Autodesk Inventor part; units mm, degrees
ref_plane "YZ Plane" through (0, 0, 0) normal (1, 0, 0) x (0, 1, 0)
ref_plane "XZ Plane" through (0, 0, 0) normal (0, 1, 0) x (-1, 0, 0)
ref_plane "XY Plane" through (0, 0, 0) normal (0, 0, 1) x (1, 0, 0)
sketch "Sketch1" plane through (0, 0, 0) normal (0, 0, 1) x (1, 0, 0)
  line L0 (-61.3765, 63.5) -> (14.8235, 63.5)
  line L1 (52.9235, 25.4) -> (52.9235, 0)
  line L2 (52.9235, 0) -> (-61.3765, 0)
  line L3 (-61.3765, 0) -> (-61.3765, 63.5)
  line L4 (52.9235, 25.4) -> (14.8235, 25.4)
  line L5 (14.8235, 25.4) -> (14.8235, 63.5)
  point P0 (0, 0)
  dimension "d0" = 38.1
  dimension "d1" = 76.2
  dimension "d2" = 38.1
  dimension "d3" = 114.3
  dimension "d4" = 63.5
  dimension "d5" = 25.4
extrude "Extrusion1" add sketch "Sketch1" along normal blind 12.7
sketch "Sketch2" plane through (0, 0, 12.7) normal (0, 0, 1) x (1, 0, 0)
  line L0 (-61.3765, 0) -> (52.9235, 0)
  line L1 (-61.3765, 63.5) -> (-61.3765, 0)
  line L2 (52.9235, 0) -> (-61.3765, 0)
  line L3 (-61.3765, 0) -> (-61.3765, 12.7)
  line L4 (-61.3765, 12.7) -> (52.9235, 12.7)
  line L5 (52.9235, 12.7) -> (52.9235, 0)
  point P0 (0, 0)
  dimension "d8" = 12.7
extrude "Extrusion2" add sketch "Sketch2" along normal blind 12.7
sketch "Sketch3" plane through (0, 0, 0) normal (0, 0, -1) x (-1, 0, 0)
  line L0 (61.3765, 63.5) -> (61.3765, 12.7)
  line L1 (-14.8235, 25.4) -> (-14.8235, 63.5)
  line L2 (61.3765, 63.5) -> (-14.8235, 63.5)
  line L3 (-14.8235, 63.5) -> (-14.8235, 38.1)
  line L4 (-14.8235, 38.1) -> (61.3765, 38.1)
  line L5 (61.3765, 38.1) -> (61.3765, 63.5)
  point P0 (0, 0)
  dimension "d11" = 25.4
extrude "Extrusion3" add sketch "Sketch3" along normal blind 25.4
Could you check a few things on this model? Use its own coordinates, in mm. A direction names the side the tool comes from. Round coordinates to 2 decimals unless told otherwise and drop trailing zeros. Write each loop counter-clockwise with the first axis right and the second up, starting at its lowest first coordinate (ties: lowest second). Pieces come first, ordered by that corner, then holes. Notation, with made-up numbers: (10, 54) -> (63, 54) arc R29 ccw to (63, 87) -> close; hole circle Ø10 at (32.25, 17). An arc over 180 degrees is marked (long way). Use a Markdown table: item, result.
1. Please list where these lines run through material, in increasing order: probe 1 along Z at (x, y) = (-38, 60); probe 2 along Z at (x, y) = (-32, 21); probe 3 along X at (y, z) = (54, 2.5).
Answer key:
| item | result |
|---|---|
| probe 1 | z = -25.4 to 12.7 |
| probe 2 | z = 0 to 12.7 |
| probe 3 | x = -61.38 to 14.82 |
2. For pin 1 Ø2 at (x, y) = (32.5, 20.5) entering from +Z; pin 2 Ø19 at (y, z) = (46, -7) entering from +X; pin 3 Ø2 at (x, z) = (4, 8.5) entering from -Y; pin 4 Ø12.5 at (x, z) = (-24, -10) entering from -Y, each with a flat end and sliding along its axis, tell me the tip position at first contact or that it passes through.
Answer key:
| item | result |
|---|---|
| pin 1 | stops at z = 12.7 |
| pin 2 | stops at x = 14.82 |
| pin 3 | stops at y = 0 |
| pin 4 | stops at y = 38.1 |
3. If we section it at A-A (x = -30): List the corners of the cut face in (y, z) for me, then the cut area to 3 significant figures.
Answer key:
| item | result |
|---|---|
| outline | (0, 0) -> (38.1, 0) -> (38.1, -25.4) -> (63.5, -25.4) -> (63.5, 12.7) -> (12.7, 12.7) -> (12.7, 25.4) -> (0, 25.4) -> close |
| area | 1,610 mm^2 |
4. Which directions (+Z, -Z, +X, -X, +Y, -Y) give clear straight access to the entire face, cutting with the end or side of a thin tool? Please do faces 1 (the face through (14.824, 48, -6)), 2 (the face through (-5, 19, 0)), 3 (the face through (-5, 6, 25.4)), 4 (the face through (-61.376, 39, 0)), 5 (the face through (-5, 12.7, 19)).
Answer key:
| item | result |
|---|---|
| face 1 | +Z, -Z, +X, +Y |
| face 2 | -Z, +X, -X, -Y |
| face 3 | +Z, +X, -X, +Y, -Y |
| face 4 | +Z, -Z, -X, +Y, -Y |
| face 5 | +Z, +X, -X, +Y |
5. We'd pull the mould along Y, two halves only. Please class faces 6 (the face through (34, 25.4, 6)), 7 (the face through (-23, 38.1, -13)), 8 (the face through (-18, 38, 12.7)): +Y half, -Y half, draft (parallel to the pull), parting line (faces both ways), or undercut.
Answer key:
| item | result |
|---|---|
| face 6 | +Y half |
| face 7 | -Y half |
| face 8 | draft |
6. If we section it at C-C (y = 34): List the corners of the cut face in (x, z) for me.
Answer key:
| item | result |
|---|---|
| outline | (-61.38, 0) -> (14.82, 0) -> (14.82, 12.7) -> (-61.38, 12.7) -> close |
7. If we section it at D-D (x = 41): List the corners of the cut face in (y, z) for me.
Answer key:
| item | result |
|---|---|
| outline | (0, 0) -> (25.4, 0) -> (25.4, 12.7) -> (12.7, 12.7) -> (12.7, 25.4) -> (0, 25.4) -> close |
8. If we section it at B-B (z = -4): List the corners of the cut face in (x, y) for me, then the cut area to 3 significant figures.
Answer key:
| item | result |
|---|---|
| outline | (-61.38, 38.1) -> (14.82, 38.1) -> (14.82, 63.5) -> (-61.38, 63.5) -> close |
| area | 1,940 mm^2 |
